Verification items for the finished model (mm, model axes). Face numbers are marked on the shaded views. A direction names the side the tool comes from. Round coordinates to 2 decimals unless told otherwise and drop trailing zeros. Loops run counter-clockwise (first coordinate to the right, second up) from the corner with the lowest first, then second, coordinate; pieces in that order, holes last. Notation, with made-up numbers: M 55.25,67.5 L 94.25,67.5 A16 ccw 94.25,79.5 Z; hole C 60,87 d3. An arc over 180 degrees is marked long. One line per item, written item: value.
from build123d import *

# Parameters (mm, degrees)
F0_W     = 500
F0_H     = 500
F1_DEPTH = 75
F2_W     = 300
F2_H     = 300
F4_W     = 100
F4_H     = 100
F6_R     = 5
F7_DEPTH = 300


with BuildPart() as f1:
    # F0 (on Top) → F1 (new body)
    with BuildSketch(Plane.XY):
        Rectangle(F0_W, F0_H)
    extrude(amount=F1_DEPTH)

    # F2 (on face) → F5 section 0
    with BuildSketch(Plane(origin=(0, 0, 0), x_dir=(1, 0, 0), z_dir=(0, 0, -1))):
        Rectangle(F2_W, F2_H)
    # F4 (on offset) → F5 section 1
    with BuildSketch(Plane(origin=(0, 0, -300), x_dir=(1, 0, 0), z_dir=(0, 0, -1))):
        Rectangle(F4_W, F4_H)
    loft()

    # F6 (on face) → F7 (cut)
    with BuildSketch(Plane(origin=(0, 0, -300), x_dir=(1, 0, 0), z_dir=(0, 0, -1))):
        Circle(F6_R)
    extrude(amount=-F7_DEPTH, mode=Mode.SUBTRACT)


solid = f1.part
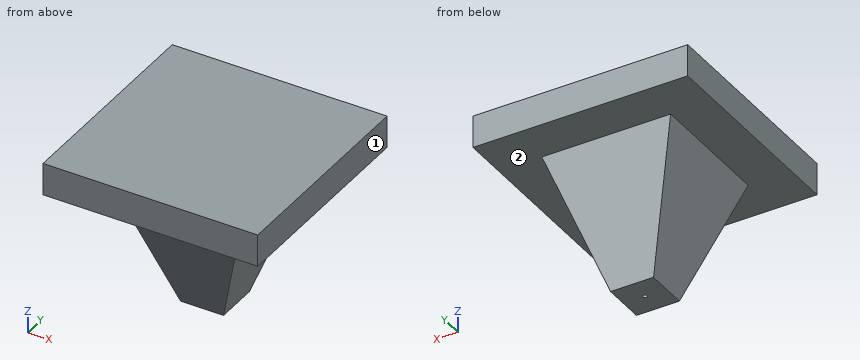
(1) Tool access check on the marked faces 1 and 2. Record the directions out of +Z, -Z, +X, -X, +Y, -Y that give a thin tool (end or side, any length) a straight path to the whole face; none if there is none.
Completed:
face 1: +Z, -Z, +X, +Y, -Y
face 2: -Z
(2) Depth check by flat-ended pin: pin 1 Ø10 at (x, z) = (51, -130) entering from -Y; pin 2 Ø8 at (x, y) = (2, 2) entering from -Z; pin 3 Ø10 at (x, z) = (-108, -31) entering from -Y; pin 4 Ø6 at (x, y) = (53, 168) entering from -Z. Enter the tip coordinate at first touch or a pass-through.
Completed:
pin 1: stops at y = -108.33
pin 2: stops at z = -300
pin 3: stops at y = -141.33
pin 4: stops at z = 0
(3) Sectioned sample at A-A on x = -158. Enter the section's corners in (y, z).
Completed:
outline: M -250,0 L 250,0 L 250,75 L -250,75 Z
(4) Thickness scan on L1, parallel to Y at x = 0, z = -207; L2, parallel to Y at x = 0, z = -62.5; L3, parallel to Z at x = -224, y = -132. Record the ranges inside material, lowest first. Write a range as from..to.
Completed:
L1: y = -81..-5, 5..81
L2: y = -129.17..-5, 5..129.17
L3: z = 0..75
